Could you check a few things on this model? Use its own coordinates, in mm. Face numbers are marked on the shaded views. A direction names the side the tool comes from. Give positions to 0.01 mm unless a question says otherwise; leave off trailing zeros. Loops run counter-clockwise (first coordinate to the right, second up) from the corner with the lowest first, then second, coordinate; pieces in that order, holes last. Notation, with made-up numbers: (-25.5, 84.5) - (-5.5, 84.5) arc R21 cw to (-5.5, 101.5) - close; hole circle Ø8 at (21.5, 15.5). An arc over 180 degrees is marked (long way). Write each question's results on one line, items separated by ' | '. Start each with the question number.
(1) For pin 1 (6 mm diameter, centred on x = 9, z = 15, fed in from +Y); pin 2 (4 mm diameter, centred on x = -17, y = 4.5, fed in from +Z); pin 3 (8 mm diameter, centred on x = -6, z = 29, fed in from -Y), each with a flat end and sliding along its axis, tell me the tip position at first contact or that it passes through.
(2) Suppose I cut it at B-B (z = 22). Please give me the cut outline in (x, y), and give its area (3 significant figures).
(3) On a 3-axis mill with a long thin cutter (end or side, diameter ignored), from which of +Z, -Z, +X, -X, +Y, -Y can I reach the whole of each face in a straight line? I mean the marked faces 1 and 2. Say none if no direction works.
(4) If we mould it in two halves opening along Z, with no side actions, what happens to the marked faces 3, 4 and 5? For each: released by +Z, released by -Z, zero draft, split by the parting line, or undercut.
(5) Suppose I cut it at D-D (z = -6). Please give me the cut outline in (x, y).
(6) I need wall thicknesses on line 1 (Y direction, x = 0, z = 36); line 2 (Z direction, x = 11, y = -8.5); line 3 (Y direction, x = 0, z = -22). Which ranges of each line are inside material? Lowest first, please.
(7) Suppose I cut it at A-A (y = 9). Count the separate pieces of the cut face and the enclosed holes in it, and give its area (3 significant figures).
from build123d import *

# Parameters (mm, degrees)
F2_T = -1.27
F4_R = 5.08


# Not quite as in the source:
# - a fillet or chamfer that OpenCascade refuses, or shapes differently, is made with other operations: its cross-section is extruded or revolved along the edge and cut away or added


with BuildPart() as f1:
    # F0 (on Front) → F1 (revolve)
    with BuildSketch(Plane.XZ):
        Polygon((0, -54.0067516267), (0, 47.3392494023), (-27.3367501795, 47.3392494023), (-27.3367501795, 14.6685000509), (-13.1127499044, 4.0005003102), (-5.7784998789, 0), (-5.7784998789, -45.7835011184), (-20.8915006369, -54.0067516267), align=None)
    revolve(axis=Axis((0, 0, -3.3337511122), (0, 0, -1)))

    # F2
    f2_openings = [f1.faces().sort_by_distance(p)[0] for p in [
        (0, 0, 47.339249),
    ]]
    offset(amount=F2_T, openings=f2_openings, kind=Kind.INTERSECTION)

    # F3: fillet of radius 5.08 on 1 edges, made by hand

    # F3_s1 → F3_t2 (revolve, cut)
    with BuildSketch(Plane.XZ):
        with BuildLine():
            ThreePointArc((-27.3371501795, 43.9787802623), (-27.0090313843, 45.775143597), (-26.0670501985, 47.3395139559))
            Line((-26.0670501985, 47.3395139559), (-26.448176769, 47.6755873252))
            ThreePointArc((-26.448176769, 47.6755873252), (-26.701900189, 47.8473859708), (-27.3367501795, 47.8473859708))
            Line((-27.3367501795, 47.8473859708), (-27.8448867481, 47.3392494023))
            ThreePointArc((-27.8448867481, 47.3392494023), (-27.8448867481, 45.6590148323), (-27.8452867481, 43.9787802623))
            Line((-27.8452867481, 43.9787802623), (-27.3371501795, 43.9787802623))
        make_face()
    revolve(axis=Axis((0, 0, 47.3392494023), (0, 0, -1)), mode=Mode.SUBTRACT)

    # F4
    f4_edges = [f1.edges().sort_by_distance(p)[0] for p in [
        (27.33675, 0, 14.6685),
        (13.11275, 0, 4.0005),
        (-20.22475, 0, 9.3345),
    ]]
    fillet(f4_edges, radius=F4_R)


solid = f1.part
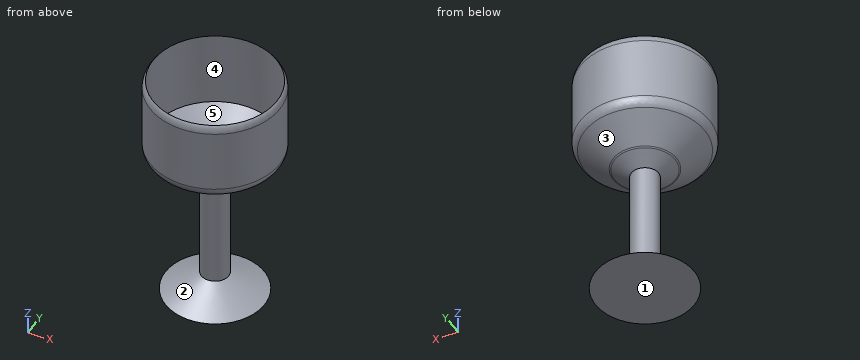
Output values:
1) pin 1: y = 26.53 | pin 2: z = 10.44 | pin 3: y = -27.26
2) outline: circle Ø54.67 at (0, 0); hole circle Ø52.13 at (0, 0) | area: 213 mm2
3) face 1: -Z, +X, -X, +Y, -Y | face 2: none
4) face 3: undercut | face 4: zero draft | face 5: released by +Z
5) outline: circle Ø11.56 at (0, 0); hole circle Ø9.02 at (0, 0)
6) line 1: -27.34 to -26.07, 26.07 to 27.34 | line 2: -54.01 to -52.74, -51.65 to -50.2, 4.59 to 6.18 | line 3: -5.78 to -4.51, 4.51 to 5.78
7) separate pieces: 2 | enclosed holes: 1 | area: 247 mm2
